Here's how the part is built. I have some questions about the finished solid (model axes, mm). A direction names the side the tool comes from. Give positions to 0.01 mm unless a question says otherwise; leave off trailing zeros. Loops run counter-clockwise (first coordinate to the right, second up) from the corner with the lowest first, then second, coordinate; pieces in that order, holes last.
Q1. Will these pins go through, and if not, where does the flat tip stop? P1, Ø1, axis at x = 19, z = 0, coming from the -Y side; P2, Ø0.9, axis at y = 2, z = 0.5, coming from the +X side; P3, Ø1.6, axis at x = 78, z = 0.5, coming from the +Y side.
Q2. If we section it at B-B (x = 8): Please give me the cut outline in (y, z).
Q3. We'd pull the mould along Y, two halves only. Please class faces 1 (the face through (35, -1, 0)), 2 (the face through (42.25, -4, 0)), 3 (the face through (43.27, -32.29, 0.02)), 4 (the face through (5.75, -7, 0)): +Y half, -Y half, draft (parallel to the pull), parting line (faces both ways), or undercut.
Q4. For faces 5 (the face through (23, 0, 0)), 6 (the face through (4, 7, 0)), 7 (the face through (3.75, -3, 0)), which set-ups out of +Z, -Z, +X, -X, +Y, -Y let a thin tool reach every point of the face, with its end or its side?
Q5. If we section it at A-A (y = -18.5): Please give me the cut outline in (x, z).
Q6. I need wall thicknesses on line 1 (X direction, y = 2, z = 0.5); line 2 (X direction, y = -2, z = 0.3); line 3 (X direction, y = -47, z = 0.85). Which ranges of each line are inside material? Lowest first, please.
from build123d import *

# Parameters (mm, degrees)
SKETCH_1_W          = 10
SKETCH_1_H          = 3
SKETCH_1_H_2        = 7
EXTRUDE_1_DEPTH     = 1.5
FILLET_1_R          = 4
EXTRUDE_2_DEPTH     = 3
CUT_EXTRUDE_1_DEPTH = 112.454026397
FILLET_2_R          = 2


with BuildPart() as part:
    # 草图1 → 凸台-拉伸1 (new, symmetric)
    with BuildSketch(Plane.XY):
        with Locations((90, -51.5)):
            Rectangle(SKETCH_1_W, SKETCH_1_H)
        Polygon((67, -50), (0, 0), (46, 0), (98, -50), align=None)
        with Locations((38, 3.5)):
            Rectangle(SKETCH_1_W, SKETCH_1_H_2)
        with Locations((8, 3.5)):
            Rectangle(SKETCH_1_W, SKETCH_1_H_2)
        with Locations((75, -51.5)):
            Rectangle(SKETCH_1_W, SKETCH_1_H)
    extrude(amount=EXTRUDE_1_DEPTH, both=True)

    # 圆角1
    fillet_1_edges = [part.edges().sort_by_distance(p)[0] for p in [
        (67, -50, 0),
        (46, 0, 0),
    ]]
    fillet(fillet_1_edges, radius=FILLET_1_R)

    # 草图5 → 凸台-拉伸2 (add)
    with BuildSketch(Plane.XY.offset(1.5)):
        with BuildLine():
            ThreePointArc((0, 0), (6.98733973, -11.453256458), (19.95552359, -14.892181783))
            Line((19.95552359, -14.892181783), (0, 0))
        make_face()
    extrude(amount=-EXTRUDE_2_DEPTH)

    # 草图2 → 切除-拉伸1 (cut, through all)
    with BuildSketch(Plane.XY.offset(1.5)):
        Polygon((72.75, -53), (72.75, -49), (70.75, -49), (70.75, -44), (72.75, -44), (72.75, -43), (77.25, -43), (77.25, -44), (79.25, -44), (79.25, -49), (77.25, -49), (77.25, -53), align=None)
        Polygon((35.75, 7), (35.75, -1), (33.75, -1), (33.75, -6), (35.75, -6), (35.75, -8), (40.25, -8), (40.25, -6), (42.25, -6), (42.25, -1), (40.25, -1), (40.25, 7), align=None)
        Polygon((10.25, 7), (5.75, 7), (5.75, -1), (3.75, -1), (3.75, -6), (5.75, -6), (5.75, -8), (10.25, -8), (10.25, -6), (12.25, -6), (12.25, -1), (10.25, -1), align=None)
    extrude(amount=-CUT_EXTRUDE_1_DEPTH, mode=Mode.SUBTRACT)

    # 草图3 → 切除-旋转3 (revolve, cut)
    with BuildSketch(Plane.XY.offset(1.5)):
        with BuildLine():
            Line((158, -63.5), (158, 177.5))
            ThreePointArc((158, 177.5), (37.5, 57), (158, -63.5))
        make_face()
    revolve(axis=Axis((158, -1021.279080972, 1.5), (0, 1, 0)), mode=Mode.SUBTRACT)

    # 圆角2
    # the kernel refuses this fillet: 2 mm, written as the material it takes off along each edge
    with BuildSketch(Plane(origin=(98, -50, -11.90231354), x_dir=(-1, 0, 0), z_dir=(0, 0, 1))) as fillet_2_piece_1:
        with BuildLine():
            CenterArc((4.385550053, -1.442307544), FILLET_2_R, 133.850179686, 92.273123028)
            Line((2.99933262, -2.883973674), (2.971608272, -2.912806996))
            Line((2.971608272, -2.912806996), (-0.027724349, -0.028833323))
            Line((-0.027724349, -0.028833323), (0, 0.04))
            ThreePointArc((0, 0.04), (1.5, 0.04), (2.972288999, 0.028846151))
            Line((2.972288999, 0.028846151), (3, 0))
        make_face()
    extrude(amount=23.80462708, mode=Mode.SUBTRACT)
    with BuildSketch(Plane(origin=(0, 0, 8.248897597), x_dir=(0.23863429141871206, -0.971109507192206, 0), z_dir=(0, 0, -1))) as fillet_2_piece_2:
        with BuildLine():
            CenterArc((2.549583536, -1.99436891), FILLET_2_R, 85.699481489, 108.106467665)
            Line((0.607364522, -2.471637493), (0.568520142, -2.481182864))
            Line((0.568520142, -2.481182864), (-0.03884438, -0.009545372))
            Line((-0.03884438, -0.009545372), (-0.00299951, 0.039887378))
            ThreePointArc((-0.00299951, 0.039887378), (1.349779519, 0.090679811), (2.702558549, 0.039887378))
            Line((2.702558549, 0.039887378), (2.699559039, 0))
        make_face()
    extrude(amount=16.497795193, mode=Mode.SUBTRACT)


solid = part.part
Check sheet entries:
1. P1: stops at y = -15.01
1. P2: stops at x = 43
1. P3: stops at y = -32.39
2. outline: (-12.16, -1.5) - (-8, -1.5) - (-8, 1.5) - (-12.16, 1.5) - close
3. face 1: undercut
3. face 2: undercut
3. face 3: -Y half
3. face 4: draft
4. face 5: +Z, -Z, +Y
4. face 6: +Z, -Z, +X, -X, +Y
4. face 7: +Z, -Z
5. outline: (24.79, -1.5) - (64.13, -1.5) arc R93.91 cw to (64.09, 1.5) - (24.79, 1.5) - close
6. line 1: x = 3 to 5.75, 10.25 to 13, 33 to 35.75, 40.25 to 43
6. line 2: x = 0.55 to 3.75, 12.25 to 33.75, 42.25 to 48.08
6. line 3: x = 62.98 to 70.75, 79.25 to 94.88
